Can you work these out from the model? Positions are in its coordinate system, mm. Give positions to 0.01 mm unless a question says otherwise; leave off trailing zeros. Loops run counter-clockwise (first coordinate to the right, second up) from the corner with the lowest first, then second, coordinate; pieces in that order, holes last. Notation, with made-up numbers: (32, 1) - (61, 1) arc R12 ccw to (61, 10) - close; hole circle Ø11 at (42.5, 74). An arc over 180 degrees is marked (long way). Answer as a JSON object with one key per item and string values. Group by question number.
Item 1: Suppose I cut it at A-A on x = -11. Write out the boundary of the cut face in (y, z).
Item 2: Thinking about a two-plate mould opening in Y: for faces 1 (the flat face through (-13.6, 1.588, 0.5)), 2 (the flat face through (-0.2, -11.5, 0.5)), 3 (the flat face through (-0.2, 11.5, 0.5)), which applies, pulls with the +Y half, pulls with the -Y half, needs draft (parallel to the pull), parting line crosses it, or undercut?
Item 3: Suppose I cut it at B-B on z = 0.6. Write out the boundary of the cut face in (x, y) (1 decimal).
Item 4: Suppose I cut it at C-C on y = 0. Write out the boundary of the cut face in (x, z), and give its area (3 significant figures).
Item 5: Please list where these lines run through material, in increasing order: L1, parallel to Y at x = -13.5, z = 0.6; L2, parallel to X at y = 1, z = 0.9; L3, parallel to X at y = -0.5, z = 0.7.
Item 6: Will this pin go through, and if not, where does the flat tip stop? pin 1 (3 mm diameter, centred on x = -12, y = -8, fed in from -Z).
from build123d import *

# Parameters (mm, degrees)
SKETCH1_W           = 31
SKETCH1_H           = 23
BOSS_EXTRUDE1_DEPTH = 1.016
CUT_EXTRUDE1_DEPTH  = 20.326982589


with BuildPart() as part:
    # Sketch1 → Boss-Extrude1 (new body)
    with BuildSketch(Plane.XY):
        Rectangle(SKETCH1_W, SKETCH1_H)
    extrude(amount=BOSS_EXTRUDE1_DEPTH)

    # Sketch2 → Cut-Extrude1 (cut, through all)
    with BuildSketch(Plane(origin=(0, 0, 0), x_dir=(-1, 0, 0), z_dir=(0, 0, -1))):
        with BuildLine():
            Line((11.825, 1.5875), (15.5, 1.5875))
            Line((15.5, 1.5875), (15.5, -1.5875))
            Line((15.5, -1.5875), (11.831296781, -1.587487512))
            ThreePointArc((11.831296781, -1.587487512), (10.237503122, -0.003148397), (11.825, 1.5875))
        make_face()
    extrude(amount=-CUT_EXTRUDE1_DEPTH, mode=Mode.SUBTRACT)


solid = part.part
Worked out:
{
 "1": {"outline": "(-11.5, 0) - (-1.36, 0) - (-1.36, 1.02) - (-11.5, 1.02) - close; (1.36, 0) - (11.5, 0) - (11.5, 1.02) - (1.36, 1.02) - close"},
 "2": {"face 1": "undercut", "face 2": "pulls with the -Y half", "face 3": "pulls with the +Y half"},
 "3": {"outline": "(-15.5, -11.5) - (15.5, -11.5) - (15.5, 11.5) - (-15.5, 11.5) - (-15.5, 1.6) - (-11.8, 1.6) arc R1.6 cw to (-11.8, -1.6) - (-15.5, -1.6) - close"},
 "4": {"outline": "(-10.24, 0) - (15.5, 0) - (15.5, 1.02) - (-10.24, 1.02) - close", "area": "26.1 mm2"},
 "5": {"L1": "y = -11.5 to -1.59, 1.59 to 11.5", "L2": "x = -10.59 to 15.5", "L3": "x = -10.32 to 15.5"},
 "6": {"pin 1": "stops at z = 0"}
}
